```python
from build123d import *

# Parameters (mm, degrees)
F0_W     = 4
F0_H     = 4
F1_DEPTH = 5
F2_T     = -1
F3_R     = 0.99999


# Not quite as in the source:
# - a fillet or chamfer is up to 0.001 mm smaller than in the source, because OpenCascade refuses the exact size


with BuildPart() as f1:
    # F0 (on Top) → F1 (new body)
    with BuildSketch(Plane.XY):
        with BuildLine():
            ThreePointArc((-2, 4.582575695), (0, 5), (2, 4.582575695))
            Line((2, 4.582575695), (2, 20))
            Line((2, 20), (-2, 20))
            Line((-2, 20), (-2, 4.582575695))
        make_face()
        with BuildLine():
            Line((2, 2), (2, 4.582575695))
            ThreePointArc((2, 4.582575695), (0, 5), (-2, 4.582575695))
            Line((-2, 4.582575695), (-2, 2))
            Line((-2, 2), (2, 2))
        make_face()
        Rectangle(F0_W, F0_H)
        with BuildLine():
            ThreePointArc((-2, -4.582575695), (0, -5), (2, -4.582575695))
            Line((2, -4.582575695), (2, -2))
            Line((2, -2), (-2, -2))
            Line((-2, -2), (-2, -4.582575695))
        make_face()
        with BuildLine():
            Line((2, -20), (2, -4.582575695))
            ThreePointArc((2, -4.582575695), (0, -5), (-2, -4.582575695))
            Line((-2, -4.582575695), (-2, -20))
            Line((-2, -20), (2, -20))
        make_face()
        with BuildLine():
            ThreePointArc((4.582575695, 2), (4.8945315647, 1.0215482184), (5, 0))
            ThreePointArc((5, 0), (4.8945315647, -1.0215482184), (4.582575695, -2))
            Line((4.582575695, -2), (20, -2))
            Line((20, -2), (20, 2))
            Line((20, 2), (4.582575695, 2))
        make_face()
        with BuildLine():
            Line((2, 2), (4.582575695, 2))
            ThreePointArc((4.582575695, 2), (3.5355339059, 3.5355339059), (2, 4.582575695))
            Line((2, 4.582575695), (2, 2))
        make_face()
        with BuildLine():
            ThreePointArc((4.582575695, -2), (4.8945315647, -1.0215482184), (5, 0))
            ThreePointArc((5, 0), (4.8945315647, 1.0215482184), (4.582575695, 2))
            Line((4.582575695, 2), (2, 2))
            Line((2, 2), (2, -2))
            Line((2, -2), (4.582575695, -2))
        make_face()
        with BuildLine():
            ThreePointArc((2, -4.582575695), (3.5355339059, -3.5355339059), (4.582575695, -2))
            Line((4.582575695, -2), (2, -2))
            Line((2, -2), (2, -4.582575695))
        make_face()
        with BuildLine():
            Line((-2, -2), (-2, 2))
            Line((-2, 2), (-4.582575695, 2))
            ThreePointArc((-4.582575695, 2), (-5, 0), (-4.582575695, -2))
            Line((-4.582575695, -2), (-2, -2))
        make_face()
        with BuildLine():
            Line((-2, 2), (-2, 4.582575695))
            ThreePointArc((-2, 4.582575695), (-3.5355339059, 3.5355339059), (-4.582575695, 2))
            Line((-4.582575695, 2), (-2, 2))
        make_face()
        with BuildLine():
            ThreePointArc((-4.582575695, -2), (-3.5355339059, -3.5355339059), (-2, -4.582575695))
            Line((-2, -4.582575695), (-2, -2))
            Line((-2, -2), (-4.582575695, -2))
        make_face()
        with BuildLine():
            ThreePointArc((-4.582575695, -2), (-5, 0), (-4.582575695, 2))
            Line((-4.582575695, 2), (-20, 2))
            Line((-20, 2), (-20, -2))
            Line((-20, -2), (-4.582575695, -2))
        make_face()
    extrude(amount=F1_DEPTH)

    # F2
    f2_openings = [f1.faces().sort_by_distance(p)[0] for p in [
        (0, 0, 5),
    ]]
    offset(amount=F2_T, openings=f2_openings, kind=Kind.INTERSECTION)

    # F3 (radius 1 in the source; OpenCascade refuses exactly that, so slightly less here)
    f3_edges = [f1.edges().sort_by_distance(p)[0] for p in [
        (0, 20, 0),
        (-2, 12.291288, 0),
        (-3.535534, 3.535534, 0),
        (-12.291288, 2, 0),
        (-20, 0, 0),
        (-12.291288, -2, 0),
        (-3.535534, -3.535534, 0),
        (-2, -12.291288, 0),
        (0, -20, 0),
        (2, -12.291288, 0),
        (3.535534, -3.535534, 0),
        (12.291288, -2, 0),
        (20, 0, 0),
        (12.291288, 2, 0),
        (3.535534, 3.535534, 0),
        (2, 12.291288, 0),
        (2, -20, 2.5),
        (-2, -20, 2.5),
        (0, -20, 5),
        (-20, 2, 2.5),
        (-20, -2, 2.5),
        (-2, 20, 2.5),
        (2, 20, 2.5),
        (20, 2, 2.5),
        (20, -2, 2.5),
    ]]
    fillet(f3_edges, radius=F3_R)


solid = f1.part
```
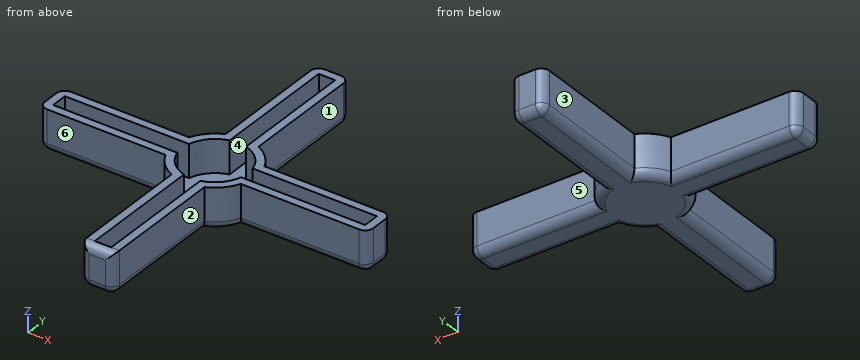
For this review, take the finished solid that the model builds, in its own axes (mm). Face numbers are marked on the shaded views. A direction names the side the tool comes from. Round coordinates to 2 decimals unless told otherwise and drop trailing zeros. Order: outer loops, then holes, each group sorted by start corner. A loop starts at its lowest first (then second) coordinate and runs counter-clockwise, first axis right, second up.
Q1. Mouldability with a two-part tool opening along Y and no side actions: class the marked faces 4, 5 and 6 as pulls with the +Y half, pulls with the -Y half, needs draft (parallel to the pull), parting line crosses it, or undercut.
Findings below:
face 4: undercut
face 5: pulls with the +Y half
face 6: pulls with the -Y half
Q2. Machinability: for the marked faces 1, 2 and 3, which of the approach directions +Z, -Z, +X, -X, +Y, -Y give a long, thin tool a straight path to every point of the face, cutting with its end or side? Answer none if there is none.
Findings below:
face 1: +Z, -Z, +X, +Y
face 2: +Z, -Z, +X, -Y
face 3: +Z, -Z, -X, +Y
Q3. Insertion check: P1, Ø2, axis at y = 13.5, z = 2, coming from the +X side; P2, Ø2, axis at y = 8.5, z = 3, coming from the -X side; P3, Ø2, axis at x = 11, z = 3, coming from the -Y side; P4, Ø1, axis at x = -10.5, y = -4, coming from the -Z side. Each pin has a flat end and moves straight along its axis. Give the tip position at first contact, or say it passes through.
Findings below:
P1: stops at x = 2
P2: stops at x = -2
P3: stops at y = -2
P4: passes through
Q4. Wall thickness on line 1 (Y direction, x = 12, z = 4.1); line 2 (Y direction, x = -4, z = 1.15): over which ranges is each line inside the solid? List them lowest first.
Findings below:
line 1: y = -2 to -1, 1 to 2
line 2: y = -3 to -1, 1 to 3
Q5. We need section A-A, the plane y = -11.5. Give the boundary of the cut face in (x, z), plus the area to 3 significant figures.
Findings below:
outline: (-2, 1) arc R1 ccw to (-1, 0) - (1, 0) arc R1 ccw to (2, 1) - (2, 5) - (1, 5) - (1, 1) - (-1, 1) - (-1, 5) - (-2, 5) - close
area: 11.6 mm2
